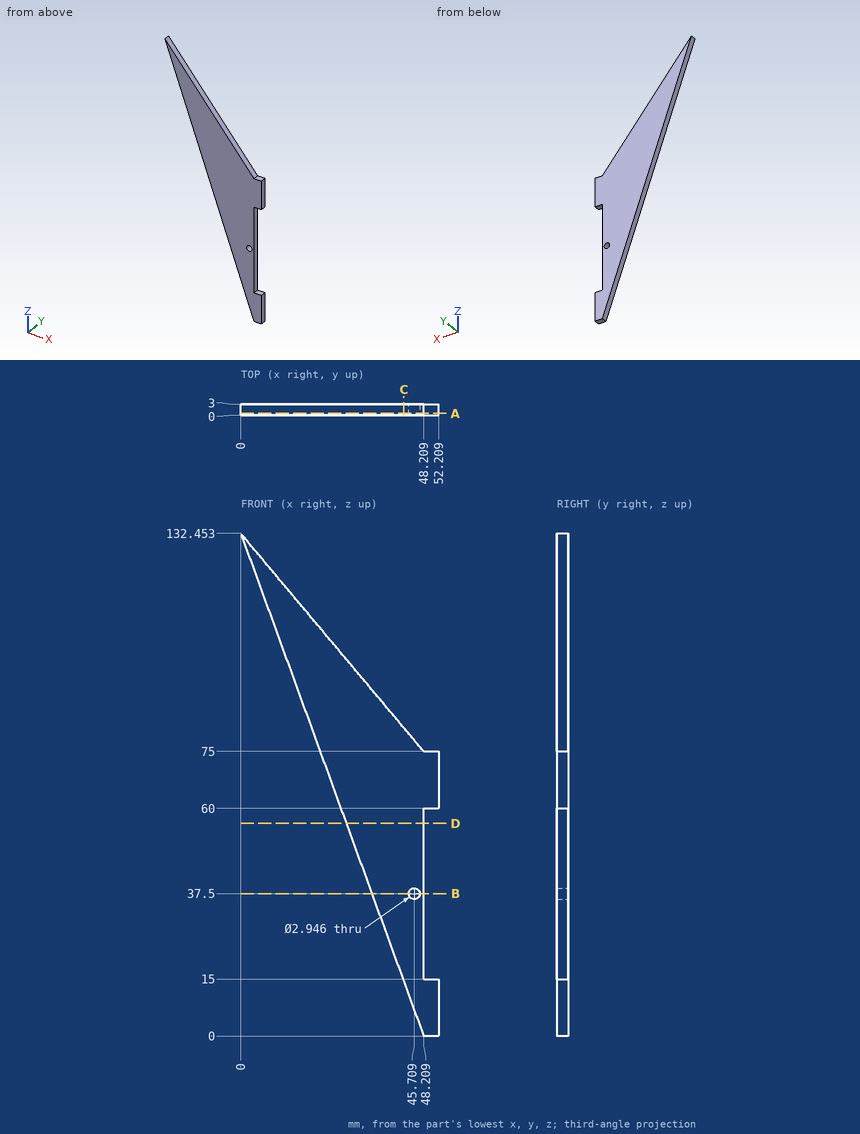
Check sheet for the drawn part. Datum: minimum x, y, z corner. Units: mm. Give positions to 0.01 mm unless a question says otherwise; leave off trailing zeros. Loops run counter-clockwise (first coordinate to the right, second up) from the corner with the lowest first, then second, coordinate; pieces in that order, holes last.
1) Sectioned sample at A-A, the plane y = 0.5. Enter the section's corners in (x, z), then the cut area to 3 significant figures.
2) Thickness scan on line 1 along Z through (x, y) = (49, 0.8); line 2 along X through (y, z) = (1.45, 11) (1 decimal); line 3 along X through (y, z) = (0.45, 120.5). Record the ranges inside material, lowest first.
3) Sectioned sample at B-B, the plane z = 37.5. Enter the section's corners in (x, y), then the cut area to 3 significant figures.
4) Sectioned sample at C-C, the plane x = 43. Enter the section's corners in (y, z).
5) Depth check by flat-ended pin: pin 1 Ø0.9 at (x, y) = (50.5, 1.5) entering from +Z; pin 2 Ø2.5 at (x, z) = (45.71, 37.5) entering from -Y; pin 3 Ø1.5 at (y, z) = (2, 30.5) entering from -X (1 decimal). Enter the tip coordinate at first touch or a pass-through.
6) Sectioned sample at D-D, the plane z = 56. Enter the section's corners in (x, y).
Answers:
1. outline: (0, 132.45) - (48.21, 0) - (52.21, 0) - (52.21, 15) - (48.21, 15) - (48.21, 60) - (52.21, 60) - (52.21, 75) - (48.21, 75) - close; hole circle Ø2.95 at (45.71, 37.5)
1. area: 1,920 mm2
2. line 1: z = 0 to 15, 60 to 75
2. line 2: x = 44.2 to 52.2
2. line 3: x = 4.35 to 10.03
3. outline: (34.56, 0) - (44.24, 0) - (44.24, 3) - (34.56, 3) - close; (47.18, 0) - (48.21, 0) - (48.21, 3) - (47.18, 3) - close
3. area: 32.1 mm2
4. outline: (0, 14.31) - (3, 14.31) - (3, 81.21) - (0, 81.21) - close
5. pin 1: stops at z = 75
5. pin 2: passes through
5. pin 3: stops at x = 36.8
6. outline: (27.83, 0) - (48.21, 0) - (48.21, 3) - (27.83, 3) - close
